Design review of the part built by this model. Coordinates are the model's own, in mm. Give positions to 0.01 mm unless a question says otherwise; leave off trailing zeros. Loops run counter-clockwise (first coordinate to the right, second up) from the corner with the lowest first, then second, coordinate; pieces in that order, holes last. Notation, with made-up numbers: (81.25, 49.25) - (95.25, 49.25) arc R11 cw to (95.25, 64.25) - close; hole circle Ø9 at (89, -5). An arc over 180 degrees is marked (long way). One line per item, written item: value. Start each with the question number.
Autodesk Inventor part; units mm, degrees
ref_plane "YZ Plane" through (0, 0, 0) normal (1, 0, 0) x (0, 1, 0)
ref_plane "XZ Plane" through (0, 0, 0) normal (0, 1, 0) x (-1, 0, 0)
ref_plane "XY Plane" through (0, 0, 0) normal (0, 0, 1) x (1, 0, 0)
sketch "Sketch1" plane through (0, 0, 0) normal (0, 1, 0) x (-1, 0, 0)
  circle A0 centre (0, 0) radius 1.5
  line L0 (0, -3) -> (-2.5981, -1.5)
  line L1 (-2.5981, -1.5) -> (-2.5981, 1.5)
  line L2 (-2.5981, 1.5) -> (0, 3)
  line L3 (0, 3) -> (2.5981, 1.5)
  line L4 (2.5981, 1.5) -> (2.5981, -1.5)
  line L5 (2.5981, -1.5) -> (0, -3)
  dimension "d0" = 3
  dimension "d1" = 3
extrude "Extrusion1" add sketch "Sketch1" along normal blind 3
(1) Take a section at B-B on y = 1.5. State the section outline as (x, z) points.
(2) Take a section at C-C on x = 1.4. State the section outline as (y, z) points.
(3) Take a section at D-D on x = -1.7. State the section outline as (y, z) points.
(4) Draft analysis for pull direction Z (two halves, no side actions). For faces 1 (the flat face through (2.598, 1, 0)), 2 (the cylindrical face through (1.5, 1.48, -0.07)), 3 (the flat face through (1.32, 1.48, 2.24)), state which applies: pulls with the +Z half, pulls with the -Z half, needs draft (parallel to the pull), parting line crosses it, or undercut.
(5) To check wall thickness, follow L1, parallel to X at y = 2.7, z = -0.05; L2, parallel to Z at x = 0.2, y = 1.4; L3, parallel to Z at x = -0.6, y = 2.3. State the ranges of each line that lie inside material, in increasing order. Write a range as from..to.
(6) Take a section at A-A on z = 0. State the section outline as (x, y) points, and give its area (3 significant figures).
(7) For pin 1 Ø2.5 at (x, z) = (0, 0) entering from +Y, flat-tipped, find the tip position at first contact; note if it passes through.
Here are the results:
1. outline: (-2.6, -1.5) - (0, -3) - (2.6, -1.5) - (2.6, 1.5) - (0, 3) - (-2.6, 1.5) - close; hole circle Ø3 at (0, 0)
2. outline: (0, -2.19) - (3, -2.19) - (3, -0.54) - (0, -0.54) - close; (0, 0.54) - (3, 0.54) - (3, 2.19) - (0, 2.19) - close
3. outline: (0, -2.02) - (3, -2.02) - (3, 2.02) - (0, 2.02) - close
4. face 1: needs draft
4. face 2: undercut
4. face 3: pulls with the +Z half
5. L1: -2.6..-1.5, 1.5..2.6
5. L2: -2.88..-1.49, 1.49..2.88
5. L3: -2.65..-1.37, 1.37..2.65
6. outline: (-2.6, 0) - (-1.5, 0) - (-1.5, 3) - (-2.6, 3) - close; (1.5, 0) - (2.6, 0) - (2.6, 3) - (1.5, 3) - close
6. area: 6.59 mm²
7. pin 1: through
